Read the model definition and answer for the solid it produces. Units are mm, in the model's axes. Face numbers are marked on the shaded views. A direction names the side the tool comes from. Coordinates: 2 decimals unless noted, no trailing zeros. Order: outer loops, then holes, each group sorted by start corner. A loop starts at its lowest first (then second) coordinate and runs counter-clockwise, first axis right, second up. Notation, with made-up numbers: M 21,-32 L 48,-32 A33 cw 48,1 Z; hole C -22,55.5 d7. An arc over 180 degrees is marked long. Use a Markdown table: item, result. Add a question column.
1) Find section A-A on z = -21. Write down the section's boundary in (x, y).
2) Find section C-C on z = 5. Write down the section's boundary in (x, y), plus the area to 3 significant figures.
3) The mould has two halves that part along X. Classify the marked faces 1, 2 and 3: released by +X, released by -X, zero draft, split by the parting line, or undercut.
4) Each of these flat-tipped pins is pushed along its axis until it touches: pin 1 Ø2.5 at (y, z) = (4, -21) entering from -X; pin 2 Ø8 at (y, z) = (5, 20) entering from -X; pin 3 Ø4.5 at (x, z) = (0, -15) entering from -Y. Where does it stop, or does it pass through?
5) Find section B-B on x = 0. Write down the section's boundary in (y, z).
6) For the marked faces 4 and 5, determine the directions among +Z, -Z, +X, -X, +Y, -Y from which every point of the face is accessible in a straight line to the end or side of a thin tool.
7) Find section D-D on y = 4.5. Count the separate pieces of the cut face and the enclosed holes in it, plus the area to 3 significant figures.
8) Find the intervals of material crossed by probe 1 along Z at (x, y) = (0, 14); probe 2 along X at (y, z) = (8.5, -6.5); probe 3 along Y at (x, z) = (4, -2), in increasing order. Write a range as [from, to].
from build123d import *

# Parameters (mm, degrees)
BOSS_EXTRUDE1_DEPTH = 25
FILLET1_R           = 3
CUT_EXTRUDE1_DEPTH  = 24
FILLET2_R           = 1
SKETCH3_R           = 2.5
CUT_EXTRUDE2_DEPTH  = 24
SKETCH4_R           = 1.5
CUT_EXTRUDE3_DEPTH  = 24
SKETCH5_R           = 2
CUT_EXTRUDE4_DEPTH  = 50


with BuildPart() as part:
    # Sketch1 → Boss-Extrude1 (new body, symmetric)
    with BuildSketch(Plane.XY):
        with BuildLine():
            Line((11.5, 0), (11.5, 11.5))
            ThreePointArc((11.5, 11.5), (10.621320344, 13.621320344), (8.5, 14.5))
            Line((8.5, 14.5), (-8.5, 14.5))
            ThreePointArc((-8.5, 14.5), (-10.621320344, 13.621320344), (-11.5, 11.5))
            Line((-11.5, 11.5), (-11.5, 0))
            Line((-11.5, 0), (-10, 0))
            Line((-10, 0), (-10, 11.5))
            ThreePointArc((-10, 11.5), (-9.560660172, 12.560660172), (-8.5, 13))
            Line((-8.5, 13), (8.5, 13))
            ThreePointArc((8.5, 13), (9.560660172, 12.560660172), (10, 11.5))
            Line((10, 11.5), (10, 0))
            Line((10, 0), (11.5, 0))
        make_face()
    extrude(amount=BOSS_EXTRUDE1_DEPTH, both=True)

    # Fillet1
    fillet1_edges = [part.edges().sort_by_distance(p)[0] for p in [
        (-10.75, 0, -25),
        (10.75, 0, -25),
        (-10.75, 0, 25),
        (10.75, 0, 25),
    ]]
    fillet(fillet1_edges, radius=FILLET1_R)

    # Sketch2 → Cut-Extrude1 (cut, through all)
    with BuildSketch(Plane(origin=(11.5, 0, 0), x_dir=(0, 0, -1), z_dir=(1, 0, 0))):
        with BuildLine():
            Line((8.5, 0), (8.5, 6))
            ThreePointArc((8.5, 6), (11, 8.5), (13.5, 6))
            Line((13.5, 6), (13.5, 0))
            Line((13.5, 0), (8.5, 0))
        make_face()
    extrude(amount=-CUT_EXTRUDE1_DEPTH, mode=Mode.SUBTRACT)

    # Fillet2
    fillet2_edges = [part.edges().sort_by_distance(p)[0] for p in [
        (-10.75, 0, -13.5),
        (10.75, 0, -13.5),
        (-10.75, 0, -8.5),
        (10.75, 0, -8.5),
    ]]
    fillet(fillet2_edges, radius=FILLET2_R)

    # Sketch3 → Cut-Extrude2 (cut, through all)
    with BuildSketch(Plane(origin=(11.5, 0, 0), x_dir=(0, 0, -1), z_dir=(1, 0, 0))):
        with Locations((-20, 5)):
            Circle(SKETCH3_R)
    extrude(amount=-CUT_EXTRUDE2_DEPTH, mode=Mode.SUBTRACT)

    # Sketch4 → Cut-Extrude3 (cut, through all)
    with BuildSketch(Plane(origin=(11.5, 0, 0), x_dir=(0, 0, -1), z_dir=(1, 0, 0))):
        with Locations((21, 4)):
            Circle(SKETCH4_R)
    extrude(amount=-CUT_EXTRUDE3_DEPTH, mode=Mode.SUBTRACT)

    # Sketch5 → Cut-Extrude4 (cut)
    with BuildSketch(Plane(origin=(0, 14.5, 0), x_dir=(1, 0, 0), z_dir=(0, 1, 0))):
        with Locations((0, 15)):
            Circle(SKETCH5_R)
        with Locations((0, -5)):
            Circle(SKETCH5_R)
    extrude(amount=-CUT_EXTRUDE4_DEPTH, mode=Mode.SUBTRACT)


solid = part.part
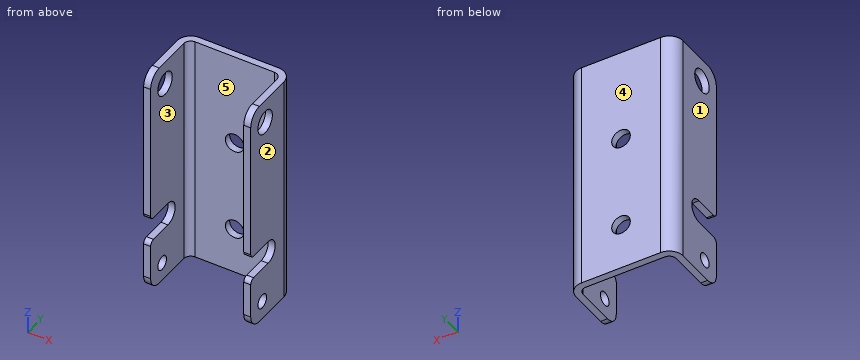
Check result:
| question | item | result |
|---|---|---|
| 1 | outline | M -11.5,0 L -10,0 L -10,2.5 L -11.5,2.5 Z; M -11.5,5.5 L -10,5.5 L -10,11.5 A1.5 cw -8.5,13 L 8.5,13 A1.5 cw 10,11.5 L 10,5.5 L 11.5,5.5 L 11.5,11.5 A3 ccw 8.5,14.5 L -8.5,14.5 A3 ccw -11.5,11.5 Z; M 10,0 L 11.5,0 L 11.5,2.5 L 10,2.5 Z |
| 2 | outline | M -11.5,0 L -10,0 L -10,11.5 A1.5 cw -8.5,13 L -2,13 L -2,14.5 L -8.5,14.5 A3 ccw -11.5,11.5 Z; M 2,13 L 8.5,13 A1.5 cw 10,11.5 L 10,0 L 11.5,0 L 11.5,11.5 A3 ccw 8.5,14.5 L 2,14.5 Z |
| 2 | area | 64.6 mm2 |
| 3 | face 1 | released by -X |
| 3 | face 2 | released by +X |
| 3 | face 3 | undercut |
| 4 | pin 1 | passes through |
| 4 | pin 2 | stops at x = -11.5 |
| 4 | pin 3 | stops at y = 13 |
| 5 | outline | M 13,-25 L 14.5,-25 L 14.5,-17 L 13,-17 Z; M 13,-13 L 14.5,-13 L 14.5,3 L 13,3 Z; M 13,7 L 14.5,7 L 14.5,25 L 13,25 Z |
| 6 | face 4 | +Z, -Z, +X, -X, +Y |
| 6 | face 5 | +Z, -Z, -Y |
| 7 | separate pieces | 8 |
| 7 | enclosed holes | 0 |
| 7 | area | 112 mm2 |
| 8 | probe 1 | z = [-25, -17], [-13, 3], [7, 25] |
| 8 | probe 2 | x = [-11.5, -10], [10, 11.5] |
| 8 | probe 3 | y = [13, 14.5] |
